Verification items for the finished model (mm, model axes). A direction names the side the tool comes from. Give positions to 0.01 mm unless a question says otherwise; leave off trailing zeros. Loops run counter-clockwise (first coordinate to the right, second up) from the corner with the lowest first, then second, coordinate; pieces in that order, holes last. Notation, with made-up numbers: (42.25, -26) - (69.25, -26) arc R25 ccw to (69.25, 10) - close; hole circle Ø4 at (76, 8). An arc over 180 degrees is marked (long way). One line per item, written item: value. Start each with the question number.
1. Mould release check, pull along X, two halves, no side actions. Record for faces 1 (the flat face through (-34.925, -18, 2)), 2 (the flat face through (18.9, 8.5, 1.6)), 3 (the flat face through (-16.03, -10.55, 1.57)), 4 (the flat face through (33, 19.05, 2)): pulls with the +X half, pulls with the -X half, needs draft (parallel to the pull), parting line crosses it, or undercut.
2. Sectioned sample at B-B (y = -13). Record the cut outline in (x, z) (1 decimal).
3. Sectioned sample at A-A (x = 26.5). Record the cut outline in (y, z) (3 decimals).
4. Gauge pin test, flat ends, axial feed: pin 1 (1 mm diameter, centred on y = 10.5, z = 1.5, fed in from -X); pin 2 (1 mm diameter, centred on x = 23.5, z = 2.5, fed in from +Y); pin 3 (1.5 mm diameter, centred on y = -11.5, z = 2, fed in from -X). Record the tip position at first contact, or that the pin passes through.
5. Sectioned sample at D-D (x = -1). Record the cut outline in (y, z) (3 decimals), plus the area to 3 significant figures.
6. Scan lines: L1, parallel to X at y = 4, z = 1.2; L2, parallel to Y at x = 25, z = 2; L3, parallel to Y at x = 32.5, z = 0.25. Record each from-to range of solid material in increasing order. Write a range as [from, to].
7. Access from +Z, -Z, +X, -X, +Y, -Y to the whole of each face (thin tool, end or side, straight path). Record for faces 5 (the flat face through (19.34, -8.74, 1.57)), 6 (the flat face through (-19.34, 8.74, 1.57)), 7 (the flat face through (0, 0, 3.175)), 8 (the flat face through (-15.584, 10.308, 1.565)).
8. Sectioned sample at C-C (z = 2.2). Record the cut outline in (x, y), plus the area to 3 significant figures.
from build123d import *

# Parameters (mm, degrees)
F1_DEPTH = 3.175


with BuildPart() as f1:
    # F0 (on Top) → F1 (new body)
    with BuildSketch(Plane.XY):
        Polygon((-2.19725e-05, 1.8082891047), (3.3151988725, -1.31744e-05), (34.9249756667, 17.2416605767), (34.9250459451, 19.05), (31.6098229194, 19.05), (31.1458046464, 18.7968994568), align=None)
        Polygon((-34.9250459451, -19.05), (-31.6098262806, -19.0500018334), (-2.29725e-05, -1.8083136201), (-3.3152438176, -1.1341e-05), (-34.925044945, -17.2416983649), align=None)
        Polygon((-34.9250449451, 17.2416983649), (-3.3152438176, -1.1341e-05), (-2.19725e-05, 1.8082891047), (-31.6098252806, 19.05), (-34.9250449451, 19.05), align=None)
        Polygon((3.3151988725, -1.31744e-05), (-2.29725e-05, -1.8083136201), (31.145784716, -18.7969359957), (31.609802849, -19.0500367955), (34.9250258747, -19.0500386289), (34.9249550549, -17.2416983648), align=None)
        Polygon((-3.3152438176, -1.1341e-05), (-2.29725e-05, -1.8083136201), (3.3151988725, -1.31744e-05), (-2.19725e-05, 1.8082891047), align=None)
    extrude(amount=F1_DEPTH)


solid = f1.part
Results are:
1. face 1: pulls with the -X half
1. face 2: pulls with the +X half
1. face 3: undercut
1. face 4: needs draft
2. outline: (-27.1, 0) - (-20.5, 0) - (-20.5, 3.2) - (-27.1, 3.2) - close; (20.5, 0) - (27.1, 0) - (27.1, 3.2) - (20.5, 3.2) - close
3. outline: (-16.263, 0) - (-12.646, 0) - (-12.646, 3.175) - (-16.263, 3.175) - close; (12.646, 0) - (16.263, 0) - (16.263, 3.175) - (12.646, 3.175) - close
4. pin 1: stops at x = -23.48
4. pin 2: stops at y = 14.9
4. pin 3: stops at x = -25.77
5. outline: (-2.354, 0) - (2.354, 0) - (2.354, 3.175) - (-2.354, 3.175) - close
5. area: 14.9 mm^2
6. L1: x = [-10.65, -4.02], [4.02, 10.65]
6. L2: y = [-15.44, -11.83], [11.83, 15.44]
6. L3: y = [-19.05, -15.92], [15.92, 19.05]
7. face 5: +Z, -Z, +X
7. face 6: +Z, -Z, -X
7. face 7: +Z, +X, -X, +Y, -Y
7. face 8: +Z, -Z, +Y
8. outline: (-34.93, -19.05) - (-31.61, -19.05) - (0, -1.81) - (31.61, -19.05) - (34.93, -19.05) - (34.92, -17.24) - (3.32, 0) - (34.92, 17.24) - (34.93, 19.05) - (31.61, 19.05) - (0, 1.81) - (-31.61, 19.05) - (-34.93, 19.05) - (-34.93, 17.24) - (-3.32, 0) - (-34.93, -17.24) - close
8. area: 481 mm^2
